```python
from build123d import *

# Parameters (mm, degrees)
F0_R     = 12.7
F1_DEPTH = 76.2
F2_R     = 12.7
F3_DEPTH = 9.525


with BuildPart() as f1:
    # F0 (on Front) → F1 (new body, symmetric)
    with BuildSketch(Plane.XZ):
        Circle(F0_R)
    extrude(amount=F1_DEPTH, both=True)

    # F2 (on face) → F3 (join)
    with BuildSketch(Plane.XZ.offset(76.2)):
        with BuildLine():
            ThreePointArc((15.1229686772, -8.7312498898), (16.867479758, -4.5196275136), (17.4625, 0))
            ThreePointArc((17.4625, 0), (16.8674797672, 4.5196274796), (15.1229687125, 8.7312498287))
            ThreePointArc((15.1229687125, 8.7312498287), (8.7312500857, 15.1229685641), (0, 17.4625))
            ThreePointArc((0, 17.4625), (-8.7312499563, 15.1229686388), (-15.1229685631, 8.7312500875))
            ThreePointArc((-15.1229685631, 8.7312500875), (-17.4625, -1.494e-07), (-15.1229684137, -8.7312503463))
            ThreePointArc((-15.1229684137, -8.7312503463), (-8.7312498116, -15.1229687224), (3.53e-08, -17.4625))
            ThreePointArc((3.53e-08, -17.4625), (8.7312500704, -15.122968573), (15.1229686772, -8.7312498898))
        make_face()
        Circle(F2_R, mode=Mode.SUBTRACT)
        Circle(F2_R)
        with BuildLine():
            ThreePointArc((0, 17.4625), (8.7312500857, 15.1229685641), (15.1229687125, 8.7312498287))
            Line((15.1229687125, 8.7312498287), (10.0819790757, 17.4625))
            Line((10.0819790757, 17.4625), (0, 17.4625))
        make_face()
        with BuildLine():
            ThreePointArc((-15.1229685631, 8.7312500875), (-8.7312499563, 15.1229686388), (0, 17.4625))
            Line((0, 17.4625), (-10.0819790757, 17.4625))
            Line((-10.0819790757, 17.4625), (-15.1229685631, 8.7312500875))
        make_face()
        with BuildLine():
            ThreePointArc((15.1229687125, 8.7312498287), (16.8674797672, 4.5196274796), (17.4625, 0))
            ThreePointArc((17.4625, 0), (16.867479758, -4.5196275136), (15.1229686772, -8.7312498898))
            Line((15.1229686772, -8.7312498898), (20.1639581514, 0))
            Line((20.1639581514, 0), (15.1229687125, 8.7312498287))
        make_face()
        with BuildLine():
            Line((10.0819790757, -17.4625), (15.1229686772, -8.7312498898))
            ThreePointArc((15.1229686772, -8.7312498898), (8.7312500704, -15.122968573), (3.53e-08, -17.4625))
            Line((3.53e-08, -17.4625), (10.0819790757, -17.4625))
        make_face()
        with BuildLine():
            Line((-10.0819790757, -17.4625), (3.53e-08, -17.4625))
            ThreePointArc((3.53e-08, -17.4625), (-8.7312498116, -15.1229687224), (-15.1229684137, -8.7312503463))
            Line((-15.1229684137, -8.7312503463), (-10.0819790757, -17.4625))
        make_face()
        with BuildLine():
            ThreePointArc((-15.1229684137, -8.7312503463), (-17.4625, -1.494e-07), (-15.1229685631, 8.7312500875))
            Line((-15.1229685631, 8.7312500875), (-20.1639581514, 0))
            Line((-20.1639581514, 0), (-15.1229684137, -8.7312503463))
        make_face()
    extrude(amount=F3_DEPTH)


solid = f1.part
```
Work out the finished part from the listing and answer in its coordinate system (mm). A direction names the side the tool comes from. Coordinates: 2 decimals unless noted, no trailing zeros. Loops run counter-clockwise (first coordinate to the right, second up) from the corner with the lowest first, then second, coordinate; pieces in that order, holes last.
1) Flat-ended cylindrical pins translate along their axes: pin 1 (4 mm diameter, centred on y = 32.5, z = -2, fed in from +X); pin 2 (3 mm diameter, centred on y = -16.5, z = -2.5, fed in from -X); pin 3 (8 mm diameter, centred on x = -15, y = -58.5, fed in from -Z). Find the tip coordinate at first contact, or state that the pin passes through.
Results:
pin 1: stops at x = 12.7
pin 2: stops at x = -12.66
pin 3: stops at z = -6.35
2) Section B-B (y = 65) is taken. Give the vertices of the cut face in (x, z).
Results:
outline: circle Ø25.4 at (0, 0)
3) Consider probe 1 along Y at (x, z) = (12.5, -4) (3 decimals); probe 2 along X at (y, z) = (32, -7.5); probe 3 along Z at (x, y) = (-9.5, 36.5). Determine where each line is inside the solid, lowest interval first.
Results:
probe 1: y = -85.725 to -76.2
probe 2: x = -10.25 to 10.25
probe 3: z = -8.43 to 8.43
4) Section A-A (x = 0) is taken. Give the vertices of the cut face in (y, z) (1 decimal), plus the area to 3 significant figures.
Results:
outline: (-85.7, -17.5) - (-76.2, -17.5) - (-76.2, -12.7) - (76.2, -12.7) - (76.2, 12.7) - (-76.2, 12.7) - (-76.2, 17.5) - (-85.7, 17.5) - close
area: 4,200 mm2
5) For faces 1 (the cylindrical face through (-2.75, -1.07, -12.4)), 2 (the flat face through (0, -81, 17.462)), determine the directions among +Z, -Z, +X, -X, +Y, -Y from which every point of the face is accessible in a straight line to the end or side of a thin tool.
Results:
face 1: +Y
face 2: +Z, +X, -X, +Y, -Y
6) Section C-C (z = 14.5) is taken. Give the vertices of the cut face in (x, y) (3 decimals).
Results:
outline: (-11.792, -85.725) - (11.792, -85.725) - (11.792, -76.2) - (-11.792, -76.2) - close
